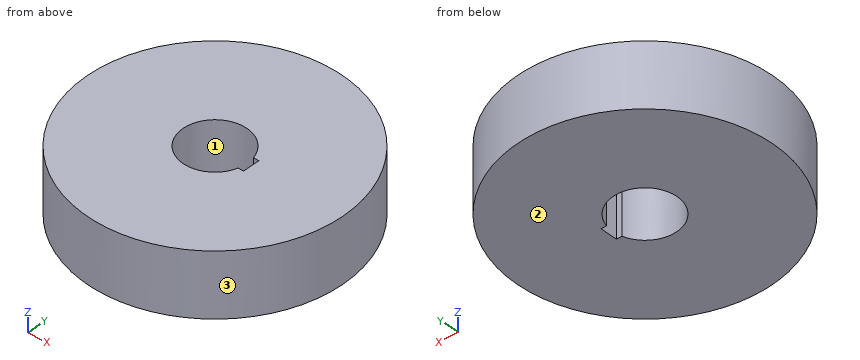
```python
from build123d import *

# Parameters (mm, degrees)
SKETCH_1_R          = 30
EXTRUDE_1_DEPTH     = 7.5
CUT_EXTRUDE_1_DEPTH = 30


with BuildPart() as part:
    # 草图1 → 凸台-拉伸1 (new, symmetric)
    with BuildSketch(Plane.XY):
        Circle(SKETCH_1_R)
    extrude(amount=EXTRUDE_1_DEPTH, both=True)

    # 草图2 → 切除-拉伸1 (cut)
    with BuildSketch(Plane.XY.offset(7.5)):
        with BuildLine():
            Line((7.228416147, 2), (8.5, 2))
            Line((8.5, 2), (8.5, -2))
            Line((8.5, -2), (7.228416147, -2))
            ThreePointArc((7.228416147, -2), (-7.5, 0), (7.228416147, 2))
        make_face()
    extrude(amount=-CUT_EXTRUDE_1_DEPTH, mode=Mode.SUBTRACT)


solid = part.part
```
Can you work these out from the model? Positions are in its coordinate system, mm. Face numbers are marked on the shaded views. Coordinates: 2 decimals unless noted, no trailing zeros. Loops run counter-clockwise (first coordinate to the right, second up) from the corner with the lowest first, then second, coordinate; pieces in that order, holes last. Notation, with made-up numbers: (7, 20.25) - (37, 20.25) arc R33 ccw to (37, 59.25) - close; hole circle Ø10 at (-15.75, 79.5). An arc over 180 degrees is marked (long way). Answer as CSV lines item,"result". Start each with the question number.
1) Suppose I cut it at A-A (y = 0). Please give me the cut outline in (x, z), plus the area to 3 significant figures.
2) Thinking about a two-plate mould opening in X: for the marked faces 1, 2 and 3, which applies, pulls with the +X half, pulls with the -X half, needs draft (parallel to the pull), parting line crosses it, or undercut?
3) I need wall thicknesses on line 1 (Y direction, x = 0, z = -2.5); line 2 (X direction, y = -3, z = -3.25). Which ranges of each line are inside material? Lowest first, please. Write a range as from..to.
4) Suppose I cut it at B-B (x = 0). Please give me the cut outline in (y, z).
5) Suppose I cut it at C-C (z = -4.75). Please give me the cut outline in (x, y), plus the area to 3 significant figures.
6) Suppose I cut it at D-D (y = -24). Please give me the cut outline in (x, z), plus the area to 3 significant figures.
7) For pin 1 (1 mm diameter, centred on x = 10.5, z = -2, fed in from +Y); pin 2 (6 mm diameter, centred on x = 7, z = -0.5, fed in from +Y); pin 3 (5 mm diameter, centred on x = -2, z = 0, fed in from -Y), each with a flat end and sliding along its axis, tell me the tip position at first contact or that it passes through.
Check result:
1,outline,"(-30, -7.5) - (-7.5, -7.5) - (-7.5, 7.5) - (-30, 7.5) - close; (8.5, -7.5) - (30, -7.5) - (30, 7.5) - (8.5, 7.5) - close"
1,area,"660 mm²"
2,face 1,"undercut"
2,face 2,"needs draft"
2,face 3,"parting line crosses it"
3,line 1,"y = -30..-7.5, 7.5..30"
3,line 2,"x = -29.85..-6.87, 6.87..29.85"
4,outline,"(-30, -7.5) - (-7.5, -7.5) - (-7.5, 7.5) - (-30, 7.5) - close; (7.5, -7.5) - (30, -7.5) - (30, 7.5) - (7.5, 7.5) - close"
5,outline,"circle Ø60 at (0, 0); hole (7.23, -2) - (8.5, -2) - (8.5, 2) - (7.23, 2) arc R7.5 ccw (long way) to start"
5,area,"2,650 mm²"
6,outline,"(-18, -7.5) - (18, -7.5) - (18, 7.5) - (-18, 7.5) - close"
6,area,"540 mm²"
7,pin 1,"stops at y = 28.28"
7,pin 2,"stops at y = 29.73"
7,pin 3,"stops at y = -30"
